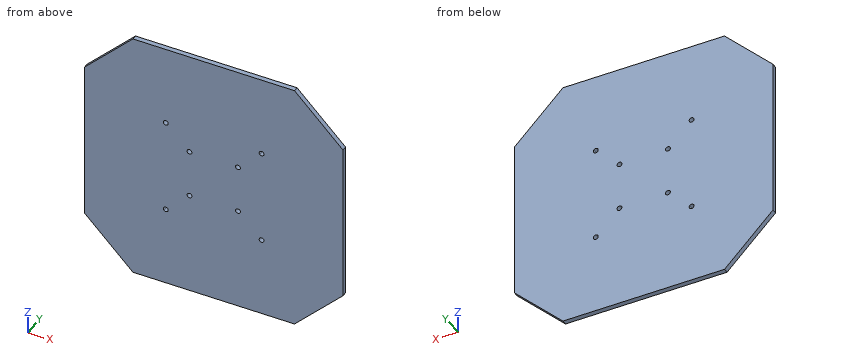
```python
from build123d import *

# Parameters (mm, degrees)
BOSS_EXTRUDE1_DEPTH = 3
SKETCH3_R           = 1.5
CUT_EXTRUDE1_DEPTH  = 10


with BuildPart() as part:
    # Sketch1 → Boss-Extrude1 (new body)
    with BuildSketch(Plane(origin=(0, 0, 0), x_dir=(1, 0, 0), z_dir=(0, 1, 0))):
        Polygon((0, 130), (30, 160), (130, 160), (160, 130), (160, 30), (130, 0), (30, 0), (0, 30), align=None)
    extrude(amount=BOSS_EXTRUDE1_DEPTH)

    # Sketch3 → Cut-Extrude1 (cut)
    with BuildSketch(Plane.XZ):
        with BuildLine():
            ThreePointArc((49.294678888, -49.294678888), (49.294678888, -51.415999231), (51.415999231, -51.415999231))
            Line((51.415999231, -51.415999231), (49.294678888, -49.294678888))
        make_face()
        with BuildLine():
            Line((49.294678888, -49.294678888), (51.415999231, -51.415999231))
            ThreePointArc((51.415999231, -51.415999231), (51.741158358, -50.929364208), (51.855339059, -50.355339059))
            ThreePointArc((51.855339059, -50.355339059), (50.929364208, -48.969519761), (49.294678888, -49.294678888))
        make_face()
        with BuildLine():
            ThreePointArc((110.705321112, -49.294678888), (108.584000769, -49.294678888), (108.584000769, -51.415999231))
            Line((108.584000769, -51.415999231), (110.705321112, -49.294678888))
        make_face()
        with BuildLine():
            Line((110.705321112, -49.294678888), (108.584000769, -51.415999231))
            ThreePointArc((108.584000769, -51.415999231), (110.218686089, -51.741158358), (111.144660941, -50.355339059))
            ThreePointArc((111.144660941, -50.355339059), (111.030480239, -49.781313911), (110.705321112, -49.294678888))
        make_face()
        with BuildLine():
            ThreePointArc((111.144660941, -109.644660941), (110.218686089, -108.258841642), (108.584000769, -108.584000769))
            Line((108.584000769, -108.584000769), (110.705321112, -110.705321112))
            ThreePointArc((110.705321112, -110.705321112), (111.030480239, -110.218686089), (111.144660941, -109.644660941))
        make_face()
        with BuildLine():
            Line((110.705321112, -110.705321112), (108.584000769, -108.584000769))
            ThreePointArc((108.584000769, -108.584000769), (108.584000769, -110.705321112), (110.705321112, -110.705321112))
        make_face()
        with BuildLine():
            ThreePointArc((51.415999231, -108.584000769), (49.294678888, -108.584000769), (49.294678888, -110.705321112))
            Line((49.294678888, -110.705321112), (51.415999231, -108.584000769))
        make_face()
        with BuildLine():
            Line((51.415999231, -108.584000769), (49.294678888, -110.705321112))
            ThreePointArc((49.294678888, -110.705321112), (50.929364208, -111.030480239), (51.855339059, -109.644660941))
            ThreePointArc((51.855339059, -109.644660941), (51.741158358, -109.070635792), (51.415999231, -108.584000769))
        make_face()
        with Locations((65, -95)):
            Circle(SKETCH3_R)
        with Locations((95, -95)):
            Circle(SKETCH3_R)
        with Locations((65, -65)):
            Circle(SKETCH3_R)
        with Locations((95, -65)):
            Circle(SKETCH3_R)
    extrude(amount=-CUT_EXTRUDE1_DEPTH, mode=Mode.SUBTRACT)


solid = part.part
```
Geometry check sheet. Reference: the model listing, model coordinates, mm. Coordinates: 2 decimals unless noted, no trailing zeros. Order: outer loops, then holes, each group sorted by start corner. A loop starts at its lowest first (then second) coordinate and runs counter-clockwise, first axis right, second up.
Item 1: Section check B-B (z = -23). Enter the section's corners in (x, y).
Item 2: Section check A-A (y = 0.6). Count the separate pieces of the cut face and the enclosed holes in it, plus the area to 3 significant figures.
Item 3: Section check C-C (x = 13.5). Enter the section's corners in (y, z), plus the area to 3 significant figures.
Item 4: Scan lines: line 1 along Z through (x, y) = (65, 0.95); line 2 along X through (y, z) = (2.4, -95); line 3 along Z through (x, y) = (29.5, 1.6). Record each from-to range of solid material in increasing order.
Check sheet entries:
1. outline: (7, 0) - (153, 0) - (153, 3) - (7, 3) - close
2. separate pieces: 1
2. enclosed holes: 8
2. area: 23,700 mm2
3. outline: (0, -143.5) - (3, -143.5) - (3, -16.5) - (0, -16.5) - close
3. area: 381 mm2
4. line 1: z = -160 to -96.5, -93.5 to -66.5, -63.5 to 0
4. line 2: x = 0 to 63.5, 66.5 to 93.5, 96.5 to 160
4. line 3: z = -159.5 to -0.5
